from build123d import *

# Parameters (mm, degrees)
ESBO_O1_R                = 20
ESBO_O1_R_2              = 1.75
RESSALTO_EXTRUS_O1_DEPTH = 3


with BuildPart() as part:
    # Esboço1 → Ressalto-extrusão1 (new body)
    with BuildSketch(Plane(origin=(0, 0, 0), x_dir=(1, 0, 0), z_dir=(0, 1, 0))):
        with Locations(Location((0, 0, 0), (0, 0, 270))):
            Circle(ESBO_O1_R)
        with Locations(Location((-8, 13.856406461, 0), (0, 0, 270))):
            Circle(ESBO_O1_R_2, mode=Mode.SUBTRACT)
        with Locations(Location((-13.856406461, 8, 0), (0, 0, 270))):
            Circle(ESBO_O1_R_2, mode=Mode.SUBTRACT)
        with Locations(Location((-16, 0, 0), (0, 0, 270))):
            Circle(ESBO_O1_R_2, mode=Mode.SUBTRACT)
        with Locations(Location((-13.856406461, -8, 0), (0, 0, 270))):
            Circle(ESBO_O1_R_2, mode=Mode.SUBTRACT)
        with Locations(Location((-8, -13.856406461, 0), (0, 0, 270))):
            Circle(ESBO_O1_R_2, mode=Mode.SUBTRACT)
        with Locations(Location((8, -13.856406461, 0), (0, 0, 270))):
            Circle(ESBO_O1_R_2, mode=Mode.SUBTRACT)
        with Locations(Location((0, -16, 0), (0, 0, 270))):
            Circle(ESBO_O1_R_2, mode=Mode.SUBTRACT)
        with Locations(Location((13.856406461, -8, 0), (0, 0, 270))):
            Circle(ESBO_O1_R_2, mode=Mode.SUBTRACT)
        with Locations(Location((16, 0, 0), (0, 0, 270))):
            Circle(ESBO_O1_R_2, mode=Mode.SUBTRACT)
        with Locations(Location((13.856406461, 8, 0), (0, 0, 270))):
            Circle(ESBO_O1_R_2, mode=Mode.SUBTRACT)
        with Locations(Location((8, 13.856406461, 0), (0, 0, 270))):
            Circle(ESBO_O1_R_2, mode=Mode.SUBTRACT)
        with Locations(Location((0, 16, 0), (0, 0, 270))):
            Circle(ESBO_O1_R_2, mode=Mode.SUBTRACT)
        with Locations(Location((0, 8, 0), (0, 0, 270))):
            Circle(ESBO_O1_R_2, mode=Mode.SUBTRACT)
        with Locations(Location((-6.92820323, -4, 0), (0, 0, 270))):
            Circle(ESBO_O1_R_2, mode=Mode.SUBTRACT)
        with Locations(Location((6.92820323, -4, 0), (0, 0, 270))):
            Circle(ESBO_O1_R_2, mode=Mode.SUBTRACT)
    extrude(amount=RESSALTO_EXTRUS_O1_DEPTH)


solid = part.part
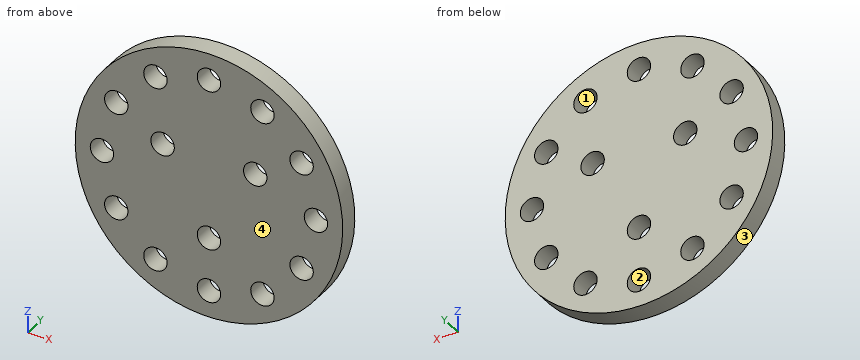
For this review, take the finished solid that the model builds, in its own axes (mm). Face numbers are marked on the shaded views. Give positions to 0.01 mm unless a question says otherwise; leave off trailing zeros. Loops run counter-clockwise (first coordinate to the right, second up) from the corner with the lowest first, then second, coordinate; pieces in that order, holes last. Notation, with made-up numbers: (7, -13) -> (15, -13) arc R15 ccw to (15, -2) -> close; hole circle Ø9 at (59.25, 85). An arc over 180 degrees is marked (long way). One line per question, with ' | ' between items.
1) We need section D-D (x = 10.5). Write out the cut boundary in (y, z).
Resolved:
outline: (0, -17.02) -> (3, -17.02) -> (3, 17.02) -> (0, 17.02) -> close
2) We need section B-B (z = -8). Write out the cut boundary in (x, y), plus the area to 3 significant figures.
Resolved:
outline: (-18.33, 0) -> (-15.61, 0) -> (-15.61, 3) -> (-18.33, 3) -> close; (-12.11, 0) -> (-1.75, 0) -> (-1.75, 3) -> (-12.11, 3) -> close; (1.75, 0) -> (12.11, 0) -> (12.11, 3) -> (1.75, 3) -> close; (15.61, 0) -> (18.33, 0) -> (18.33, 3) -> (15.61, 3) -> close | area: 78.5 mm2
3) We need section C-C (y = 1.4). Give the number of separate pieces and of enclosed holes in the cut face, plus the area to 3 significant figures.
Resolved:
separate pieces: 1 | enclosed holes: 15 | area: 1,110 mm2
4) The part is to be moulded in two halves that separate along Z. For the marked faces 1, 2, 3 and 4, say which applies: +Z half, -Z half, draft (parallel to the pull), parting line (faces both ways), or undercut.
Resolved:
face 1: undercut | face 2: undercut | face 3: parting line | face 4: draft
5) We need section A-A (z = 4). Write out the cut boundary in (x, y).
Resolved:
outline: (-19.6, 0) -> (-8.68, 0) -> (-8.68, 3) -> (-19.6, 3) -> close; (-5.18, 0) -> (5.18, 0) -> (5.18, 3) -> (-5.18, 3) -> close; (8.68, 0) -> (19.6, 0) -> (19.6, 3) -> (8.68, 3) -> close
6) Insertion check: pin 1 Ø3 at (x, z) = (0, 16) entering from +Y; pin 2 Ø1.5 at (x, y) = (-2.5, 2) entering from +Z; pin 3 Ø1 at (y, z) = (1.5, 12) entering from -X. Each pin has a flat end and moves straight along its axis. Give the tip position at first contact, or say it passes through.
Resolved:
pin 1: passes through | pin 2: stops at z = 19.92 | pin 3: stops at x = -16.36
7) To check wall thickness, follow probe 1 along X at (y, z) = (2.3, 0); probe 2 along X at (y, z) = (0.6, 7.5); probe 3 along Z at (x, y) = (-12.5, 0.65). State the ranges of each line that lie inside material, in increasing order.
Resolved:
probe 1: x = -20 to -17.75, -14.25 to 14.25, 17.75 to 20 | probe 2: x = -18.54 to -15.53, -12.18 to 12.18, 15.53 to 18.54 | probe 3: z = -15.61 to -9.11, -6.89 to 6.89, 9.11 to 15.61
